For this review, take the finished solid that the model builds, in its own axes (mm). Face numbers are marked on the shaded views. A direction names the side the tool comes from. Round coordinates to 2 decimals unless told otherwise and drop trailing zeros. Write each loop counter-clockwise with the first axis right and the second up, starting at its lowest first coordinate (ties: lowest second). Pieces come first, ordered by that corner, then holes. Notation, with made-up numbers: M -32,51.5 L -21,51.5 A23 cw -21,89.5 Z; hole C 76.25,-39.5 d10. An arc over 180 degrees is marked long. Answer in a Markdown table with one row per item.
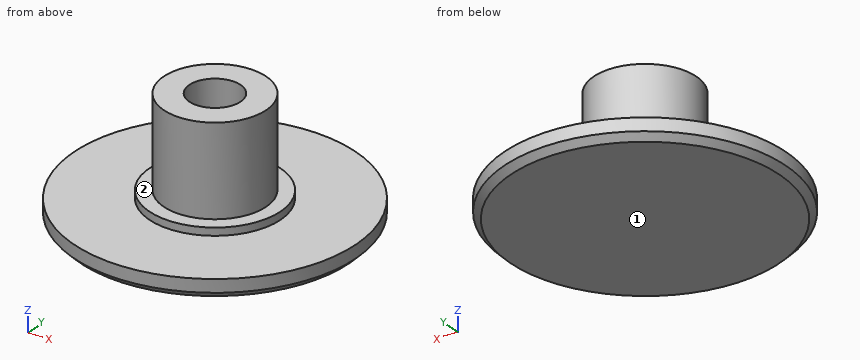
```python
from build123d import *

# Parameters (mm, degrees)
F0_R     = 11
F1_DEPTH = 1.5
F2_R     = 5.125
F3_DEPTH = 0.6
F4_R     = 4
F5_DEPTH = 7
F6_R     = 2
F7_DEPTH = 7
F8_SIZE  = 0.5


with BuildPart() as f1:
    # F0 (on Top) → F1 (new body)
    with BuildSketch(Plane.XY):
        Circle(F0_R)
    extrude(amount=F1_DEPTH)

    # F2 (on face) → F3 (join)
    with BuildSketch(Plane.XY.offset(1.5)):
        Circle(F2_R)
    extrude(amount=F3_DEPTH)

    # F4 (on face) → F5 (join)
    with BuildSketch(Plane.XY.offset(2.1)):
        Circle(F4_R)
    extrude(amount=F5_DEPTH)

    # F6 (on face) → F7 (cut, through all)
    with BuildSketch(Plane.XY.offset(9.1)):
        Circle(F6_R)
    extrude(amount=-F7_DEPTH, mode=Mode.SUBTRACT)

    # F8
    f8_edges = [f1.edges().sort_by_distance(p)[0] for p in [
        (-11, 0, 0),
    ]]
    chamfer(f8_edges, length=F8_SIZE)


solid = f1.part
```
Q1. Machinability: for the marked faces 1 and 2, which of the approach directions +Z, -Z, +X, -X, +Y, -Y give a long, thin tool a straight path to every point of the face, cutting with its end or side? Answer none if there is none.
Found:
| item | result |
|---|---|
| face 1 | -Z, +X, -X, +Y, -Y |
| face 2 | +Z |
Q2. Insertion check: P1, Ø2.5, axis at x = 0, y = 0, coming from the +Z side; P2, Ø5, axis at x = -4, y = -9, coming from the +Z side; P3, Ø4, axis at y = -2, z = 4.5, coming from the +X side. Each pin has a flat end and moves straight along its axis. Give the tip position at first contact, or say it passes through.
Found:
| item | result |
|---|---|
| P1 | z = 2.1 |
| P2 | z = 1.5 |
| P3 | x = 4 |
Q3. Take a section at A-A (x = 0). State the section outline as (y, z) points (3 decimals), then the cut area to 3 significant figures.
Found:
| item | result |
|---|---|
| outline | M -11,0.5 L -10.5,0 L 10.5,0 L 11,0.5 L 11,1.5 L 5.125,1.5 L 5.125,2.1 L 4,2.1 L 4,9.1 L 2,9.1 L 2,2.1 L -2,2.1 L -2,9.1 L -4,9.1 L -4,2.1 L -5.125,2.1 L -5.125,1.5 L -11,1.5 Z |
| area | 66.9 mm² |
Q4. For probe 1 along Y at (x, z) = (0, 7.75); probe 2 along Z at (x, y) = (-5.75, 3.5); probe 3 along Z at (x, y) = (5, -0.25), list the stretches that pass through material, from the lowest coordinate up.
Found:
| item | result |
|---|---|
| probe 1 | -4 to -2, 2 to 4 |
| probe 2 | 0 to 1.5 |
| probe 3 | 0 to 2.1 |
Q5. Take a section at B-B (z = 8). State the section outline as (x, y) points, then the cut area to 3 significant figures.
Found:
| item | result |
|---|---|
| outline | C 0,0 d8; hole C 0,0 d4 |
| area | 37.7 mm² |
